Work out the finished part from the listing and answer in its coordinate system (mm). A direction names the side the tool comes from. Coordinates: 2 decimals unless noted, no trailing zeros. Write each loop counter-clockwise with the first axis right and the second up, starting at its lowest first coordinate (ties: lowest second). Pieces come first, ordered by that corner, then holes. Notation, with made-up numbers: (62, -23) - (82, -23) arc R7 ccw to (82, -15) - close; hole circle Ø8 at (-7.75, 86). An arc over 180 degrees is marked (long way). One line per item, written item: value.
```python
from build123d import *

# Parameters (mm, degrees)
F0_R     = 6
F1_DEPTH = 10


with BuildPart() as f1:
    # F0 (on Front) → F1 (new body)
    with BuildSketch(Plane.XZ):
        with BuildLine():
            Line((100, 0), (27.078551, 152.913251))
            ThreePointArc((27.078551, 152.913251), (0, 170), (-27.078551, 152.913251))
            Line((-27.078551, 152.913251), (-100, 0))
            Line((-100, 0), (-125, 0))
            Line((-125, 0), (-125, -10))
            Line((-125, -10), (125, -10))
            Line((125, -10), (125, 0))
            Line((125, 0), (100, 0))
        make_face()
        with Locations((0, 140)):
            Circle(F0_R, mode=Mode.SUBTRACT)
    extrude(amount=F1_DEPTH)


solid = f1.part
```
Item 1: Section C-C, the plane z = 140 is taken. Determine the outline of the cut face in (x, y), then the cut area to 3 significant figures.
Evaluation:
outline: (-33.24, -10) - (-6, -10) - (-6, 0) - (-33.24, 0) - close; (6, -10) - (33.24, -10) - (33.24, 0) - (6, 0) - close
area: 545 mm2
Item 2: Given pin 1 (5 mm diameter, centred on x = 112, y = -5.5, fed in from +Z); pin 2 (5 mm diameter, centred on y = -7, z = 110, fed in from -X); pin 3 (15.5 mm diameter, centred on x = 0, z = 140, fed in from +Y); pin 4 (1 mm diameter, centred on y = -6, z = 109, fed in from +X), each flat-ended and moving along its own axis, determine where each tip first touches the part or whether it passes through.
Evaluation:
pin 1: stops at z = 0
pin 2: stops at x = -48.74
pin 3: stops at y = 0
pin 4: stops at x = 48.26
Item 3: Section B-B, the plane y = -5 is taken. Determine the outline of the cut face in (x, z), then the cut area to 3 significant figures.
Evaluation:
outline: (-125, -10) - (125, -10) - (125, 0) - (100, 0) - (27.08, 152.91) arc R30 ccw to (-27.08, 152.91) - (-100, 0) - (-125, 0) - close; hole circle Ø12 at (0, 140)
area: 22,500 mm2
Item 4: Consider probe 1 along Z at (x, y) = (-103, -1.5); probe 2 along Z at (x, y) = (9, -4); probe 3 along X at (y, z) = (-5.5, 136). Determine where each line is inside the solid, lowest interval first.
Evaluation:
probe 1: z = -10 to 0
probe 2: z = -10 to 168.62
probe 3: x = -35.14 to -4.47, 4.47 to 35.14
Item 5: Determine the mould class of faces 1 (the face through (-1.301, -4.93, 134.143)), 2 (the face through (-125, -5, -5)), 3 (the face through (-2, -5, -10)) for opening direction X: +X half, -X half, draft (parallel to the pull), parting line (faces both ways), or undercut.
Evaluation:
face 1: undercut
face 2: -X half
face 3: draft
Item 6: Section A-A, the plane x = 0 is taken. Determine the outline of the cut face in (y, z).
Evaluation:
outline: (-10, -10) - (0, -10) - (0, 134) - (-10, 134) - close; (-10, 146) - (0, 146) - (0, 170) - (-10, 170) - close
Item 7: Section D-D, the plane z = 115 is taken. Determine the outline of the cut face in (x, y).
Evaluation:
outline: (-45.16, -10) - (45.16, -10) - (45.16, 0) - (-45.16, 0) - close
Item 8: Which of the six approach directions +Z, -Z, +X, -X, +Y, -Y give full straight-line access (tool end or side, diameter ignored) to faces 4 (the face through (-112, -5, 0)), 5 (the face through (-2, -10, 61)), 6 (the face through (113, -5, 0))?
Evaluation:
face 4: +Z, -X, +Y, -Y
face 5: +Z, -Z, +X, -X, -Y
face 6: +Z, +X, +Y, -Y
